```python
from build123d import *

# Parameters (mm, degrees)
SKETCH1_W                   = 88
SKETCH1_H                   = 211
BOSS_EXTRUDE1_DEPTH         = 2
CUT_EXTRUDE2_DEPTH          = 2
SKETCH4_R                   = 5
CUT_EXTRUDE3_DEPTH          = 3
FILLET2_R                   = 3
SKETCH23_W                  = 2
SKETCH23_H                  = 211
SKETCH23_W_2                = 2.150374681
CUT_EXTRUDE5_DEPTH          = 10
SKETCH29_W                  = 5.911493913
SKETCH29_H                  = 211
SKETCH29_W_2                = 4.036537762
CUT_EXTRUDE10_DEPTH         = 2
F_5_0MM_DOWEL_HOLE1_D       = 5
TAP_DRILL_FOR_M3X0_5_TAP1_D = 2.5


with BuildPart() as part:
    # Sketch1 → Boss-Extrude1 (new body)
    with BuildSketch(Plane.XY):
        with Locations((44, 105.5)):
            Rectangle(SKETCH1_W, SKETCH1_H)
    extrude(amount=BOSS_EXTRUDE1_DEPTH)

    # Sketch3 → Cut-Extrude2 (cut)
    with BuildSketch(Plane.XY.offset(2)):
        Polygon((73, 133.88804004), (50, 147.167096231), (50, 115.5), (73, 115.5), align=None)
        Polygon((38, 115.5), (38, 147.167096231), (15, 133.88804004), (15, 115.5), align=None)
        Polygon((15, 143.125644347), (36, 155.25), (15, 167.374355653), align=None)
        Polygon((73, 143.125644347), (73, 167.374355653), (52, 155.25), align=None)
        Polygon((73, 196), (50, 196), (50, 163.332903769), (73, 176.61195996), align=None)
        Polygon((38, 163.332903769), (38, 196), (15, 196), (15, 176.61195996), align=None)
    cut_extrude2 = extrude(amount=-CUT_EXTRUDE2_DEPTH, mode=Mode.SUBTRACT)

    # Sketch4 → Cut-Extrude3 (cut, through all)
    with BuildSketch(Plane.XY.offset(2)):
        with Locations((44, 155.25)):
            Circle(SKETCH4_R)
    cut_extrude3 = extrude(amount=-CUT_EXTRUDE3_DEPTH, mode=Mode.SUBTRACT)

    # Mirror2: Cut-Extrude2, Cut-Extrude3 across plane
    add(cut_extrude2.mirror(Plane.ZX.offset(105.5)), mode=Mode.SUBTRACT)
    add(cut_extrude3.mirror(Plane.ZX.offset(105.5)), mode=Mode.SUBTRACT)

    # Fillet2
    fillet2_edges = [part.edges().sort_by_distance(p)[0] for p in [
        (36, 55.75, 1),
        (15, 43.625644347, 1),
        (15, 67.874355653, 1),
        (38, 95.5, 1),
        (38, 63.832903769, 1),
        (15, 77.11195996, 1),
        (15, 95.5, 1),
        (73, 15, 1),
        (50, 15, 1),
        (50, 47.667096231, 1),
        (73, 34.38804004, 1),
        (73, 43.625644347, 1),
        (52, 55.75, 1),
        (73, 67.874355653, 1),
        (15, 15, 1),
        (15, 34.38804004, 1),
        (38, 47.667096231, 1),
        (38, 15, 1),
        (73, 77.11195996, 1),
        (50, 63.832903769, 1),
        (50, 95.5, 1),
        (73, 95.5, 1),
        (15, 167.374355653, 1),
        (36, 155.25, 1),
        (15, 143.125644347, 1),
        (38, 147.167096231, 1),
        (38, 115.5, 1),
        (15, 115.5, 1),
        (15, 133.88804004, 1),
        (50, 196, 1),
        (73, 196, 1),
        (73, 176.61195996, 1),
        (50, 163.332903769, 1),
        (52, 155.25, 1),
        (73, 167.374355653, 1),
        (73, 143.125644347, 1),
        (15, 176.61195996, 1),
        (15, 196, 1),
        (38, 196, 1),
        (38, 163.332903769, 1),
        (50, 147.167096231, 1),
        (73, 133.88804004, 1),
        (73, 115.5, 1),
        (50, 115.5, 1),
    ]]
    fillet(fillet2_edges, radius=FILLET2_R)

    # Sketch23 → Cut-Extrude5 (cut)
    with BuildSketch(Plane.XY.offset(2)):
        with Locations((87, 105.5)):
            Rectangle(SKETCH23_W, SKETCH23_H)
        with Locations((1.075187341, 105.5)):
            Rectangle(SKETCH23_W_2, SKETCH23_H)
    extrude(amount=-CUT_EXTRUDE5_DEPTH, mode=Mode.SUBTRACT)

    # Sketch29 → Cut-Extrude10 (cut)
    with BuildSketch(Plane(origin=(0, 0, 0), x_dir=(-1, 0, 0), z_dir=(0, 0, -1))):
        with Locations((-1.044253043, 105.5)):
            Rectangle(SKETCH29_W, SKETCH29_H)
        with Locations((-86.018268881, 105.5)):
            Rectangle(SKETCH29_W_2, SKETCH29_H)
    extrude(amount=-CUT_EXTRUDE10_DEPTH, mode=Mode.SUBTRACT)

    # Ø5.0mm Dowel Hole1 (through all)
    with Locations(Plane.XY.offset(2)):
        with Locations((24, 205), (64, 205), (9, 184), (79, 184), (9, 135), (79, 135), (79, 109.2), (9, 109.2), (9, 79.2), (79, 79.2), (79, 59.2), (9, 59.2), (9, 33.2), (79, 33.2), (64, 6), (24, 6)):
            Hole(F_5_0MM_DOWEL_HOLE1_D / 2)

    # Tap Drill for M3x0.5 Tap1 (through all)
    with Locations(Plane.XY.offset(2)):
        with Locations((9, 23), (79, 23), (9, 196), (79, 196)):
            Hole(TAP_DRILL_FOR_M3X0_5_TAP1_D / 2)


solid = part.part
```
Geometry: final body of the model. Coordinates: model frame, mm. A direction names the side the tool comes from. Give positions to 0.01 mm unless a question says otherwise; leave off trailing zeros. Write each loop counter-clockwise with the first axis right and the second up, starting at its lowest first coordinate (ties: lowest second). Pieces come first, ordered by that corner, then holes.
1. Section query B-B, the plane y = 122. Return loops of the section in (x, z).
2. Line query: probe 1 along X at (y, z) = (83.5, 1.4); probe 2 along Y at (x, z) = (35.5, 1.45); probe 3 along X at (y, z) = (155.5, 1.4). Output: solid intervals per line, ascending.
3. Section query C-C, the plane y = 184. Return loops of the section in (x, z).
4. Pin query (flat end, axial travel): P1, Ø3, axis at x = 64, y = 6, coming from the +Z side. Return the tip coordinate at first contact, or that it passes through.
5. Section query A-A, the plane x = 44. Return loops of the section in (y, z), then the cut area to 3 significant figures.
6. Draft query along X for faces 3 (the flat face through (62.88, 40.23, 1.01)), 4 (the flat face through (43, 107, 0)), 5 (the cylindrical face through (40.315, 52.371, 1.014)). Return one class per face: released by +X, released by -X, zero draft, split by the parting line, or undercut.
7. Reachability of faces 1 (the flat face through (25.584, 49.736, 1.014)), 2 (the flat face through (43, 107, 2)) from +Z, -Z, +X, -X, +Y, -Y: full face, straight path, thin tool, end or side. Return the list, or none.
8. Section query D-D, the plane z = 0.4. Count the separate pieces of the cut face and the enclosed holes in it, then the cut area to 3 significant figures.
Computed:
1. outline: (4, 0) - (15, 0) - (15, 2) - (4, 2) - close; (38, 0) - (50, 0) - (50, 2) - (38, 2) - close; (73, 0) - (84, 0) - (84, 2) - (73, 2) - close
2. probe 1: x = 4 to 15, 38 to 50, 73 to 84
2. probe 2: y = 0 to 15.04, 45.43 to 66.07, 95.46 to 115.54, 144.93 to 165.57, 195.96 to 211
2. probe 3: x = 4 to 15, 32.99 to 39.01, 48.99 to 55.01, 73 to 84
3. outline: (4, 0) - (6.5, 0) - (6.5, 2) - (4, 2) - close; (11.5, 0) - (15, 0) - (15, 2) - (11.5, 2) - close; (38, 0) - (50, 0) - (50, 2) - (38, 2) - close; (73, 0) - (76.5, 0) - (76.5, 2) - (73, 2) - close; (81.5, 0) - (84, 0) - (84, 2) - (81.5, 2) - close
4. P1: passes through
5. outline: (0, 0) - (50.75, 0) - (50.75, 2) - (0, 2) - close; (60.75, 0) - (150.25, 0) - (150.25, 2) - (60.75, 2) - close; (160.25, 0) - (211, 0) - (211, 2) - (160.25, 2) - close
5. area: 382 mm2
6. face 3: undercut
6. face 4: zero draft
6. face 5: undercut
7. face 1: +Z, -Z
7. face 2: +Z, +X, -X, +Y, -Y
8. separate pieces: 1
8. enclosed holes: 34
8. area: 10,800 mm2
